from build123d import *

# Parameters (mm, degrees)
F0_W      = 150
F0_H      = 19
F1_DEPTH  = 50
F3_DEPTH  = 19
F4_W      = 79
F4_H      = 30
F5_DEPTH  = 35.4
F8_DEPTH  = 30
F9_W      = 54.530326277
F9_H      = 30
F10_DEPTH = 2
F12_DEPTH = 13
F14_DEPTH = 13
F15_R     = 5
F16_DEPTH = 13
F18_DEPTH = 13
F19_R     = 10
F20_DEPTH = 19
F21_DEPTH = 19


with BuildPart() as f1:
    # F0 (on Front) → F1 (new body)
    with BuildSketch(Plane.XZ):
        with Locations((0, 1.0748035961)):
            Rectangle(F0_W, F0_H)
    extrude(amount=F1_DEPTH)

    # F2 (on face) → F3 (join)
    with BuildSketch(Plane.XY.offset(10.5748035961)):
        with BuildLine():
            Line((-75, -50), (-75, 0))
            ThreePointArc((-75, 0), (-100, -25), (-75, -50))
        make_face()
        with BuildLine():
            ThreePointArc((75, -50), (100, -25), (75, 0))
            Line((75, 0), (75, -50))
        make_face()
    extrude(amount=-F3_DEPTH)

    # F4 (on Top) → F5 (join)
    with BuildSketch(Plane.XY):
        with Locations((3.0394736677, -23.589033746)):
            Rectangle(F4_W, F4_H)
    extrude(amount=F5_DEPTH)

    # F7 (on face) → F8 (cut)
    with BuildSketch(Plane.XZ.offset(38.589033746)):
        with BuildLine():
            Line((31.6433943808, 35.2142751217), (-23.7523913383, 34.8830260336))
            ThreePointArc((-23.7523913383, 34.8830260336), (4.0825457385, 12.1303321123), (31.6433943808, 35.2142751217))
        make_face()
    extrude(amount=-F8_DEPTH, mode=Mode.SUBTRACT)

    # F9 (on face) → F10 (cut)
    with BuildSketch(Plane.XY.offset(35.4)):
        with Locations((4.4306721538, -23.589033746)):
            Rectangle(F9_W, F9_H)
    extrude(amount=-F10_DEPTH, mode=Mode.SUBTRACT)

    # F11 (on face) → F12 (join)
    with BuildSketch(Plane(origin=(-36.4605263323, 0, 0), x_dir=(0, -1, 0), z_dir=(-1, 0, 0))):
        with BuildLine():
            Line((8.589033746, 35.4), (38.589033746, 35.4))
            ThreePointArc((38.589033746, 35.4), (23.589033746, 50.4), (8.589033746, 35.4))
        make_face()
    extrude(amount=-F12_DEPTH)

    # F13 (on face) → F14 (join)
    with BuildSketch(Plane.YZ.offset(42.5394736677)):
        with BuildLine():
            Line((-38.589033746, 35.4), (-8.589033746, 35.4))
            ThreePointArc((-8.589033746, 35.4), (-23.589033746, 50.4), (-38.589033746, 35.4))
        make_face()
    extrude(amount=-F14_DEPTH)

    # F15 (on face) → F16 (cut)
    with BuildSketch(Plane.YZ.offset(42.5394736677)):
        with Locations((-23.6123930663, 39.6284162998)):
            Circle(F15_R)
    extrude(amount=-F16_DEPTH, mode=Mode.SUBTRACT)

    # F17 (on face) → F18 (cut)
    with BuildSketch(Plane.YZ.offset(-23.4605263323)):
        with BuildLine():
            Line((-21.2145990318, 35.4), (-26.3218262607, 35.4))
            ThreePointArc((-26.3218262607, 35.4), (-23.7682126462, 34.6987274289), (-21.2145990318, 35.4))
        make_face()
        with BuildLine():
            ThreePointArc((-21.2145990318, 35.4), (-19.4226362707, 37.2256795192), (-18.7682126462, 39.6987274289))
            ThreePointArc((-18.7682126462, 39.6987274289), (-26.241260556, 44.0443038045), (-26.3218262607, 35.4))
            Line((-26.3218262607, 35.4), (-21.2145990318, 35.4))
        make_face()
    extrude(amount=-F18_DEPTH, mode=Mode.SUBTRACT)

    # F19 (on face) → F20 (cut)
    with BuildSketch(Plane.XY.offset(10.5748035961)):
        with Locations((-84.4740969445, -25.0065810978)):
            Circle(F19_R)
    extrude(amount=-F20_DEPTH, mode=Mode.SUBTRACT)

    # F19 (on face) → F21 (cut)
    with BuildSketch(Plane.XY.offset(10.5748035961)):
        with Locations((-84.4740969445, -25.0065810978)):
            Circle(F19_R)
        with Locations((84.4793568792, -25.0065810978)):
            Circle(F19_R)
    extrude(amount=-F21_DEPTH, mode=Mode.SUBTRACT)


solid = f1.part
Verification items for the finished model (mm, model axes). A direction names the side the tool comes from. Coordinates: 2 decimals unless noted, no trailing zeros. Order: outer loops, then holes, each group sorted by start corner. A loop starts at its lowest first (then second) coordinate and runs counter-clockwise, first axis right, second up. Notation, with made-up numbers: M 64.25,81.25 L 104.25,81.25 A15 cw 104.25,100.25 Z; hole C 58.5,86 d8. An arc over 180 degrees is marked long. Return JSON: item names as keys, results as strings.
1) Thickness scan on L1, parallel to X at y = -33, z = -2.5; L2, parallel to X at y = -24, z = -0.5; L3, parallel to X at y = -38, z = 39. Record the ranges inside material, lowest first. Write a range as [from, to].
Answer list:
{"L1": "[-98.69, -90.48], [-78.47, 78.47], [90.49, 98.69]", "L2": "[-99.98, -94.42], [-74.52, 74.53], [94.43, 99.98]", "L3": "[-36.46, -23.46], [29.54, 42.54]"}
2) Gauge pin test, flat ends, axial feed: pin 1 (0.5 mm diameter, centred on x = 31.5, y = -25, fed in from +Z) (3 decimals); pin 2 (12 mm diameter, centred on x = 84.48, y = -25.01, fed in from +Z); pin 3 (1.5 mm diameter, centred on y = -18, z = 43.5, fed in from -X); pin 4 (13 mm diameter, centred on y = -23.61, z = 39.63, fed in from +X). Record the tip position at first contact, or that the pin passes through.
Answer list:
{"pin 1": "z = 50.355", "pin 2": "through", "pin 3": "x = -36.46", "pin 4": "x = 42.54"}
3) Cross-section at C-C, the plane x = 83. Record the boundary of the cut face in (y, z), and give its area (3 significant figures).
Answer list:
{"outline": "M -48.69,-8.43 L -34.9,-8.43 L -34.9,10.57 L -48.69,10.57 Z; M -15.12,-8.43 L -1.31,-8.43 L -1.31,10.57 L -15.12,10.57 Z", "area": "524 mm2"}
4) Release check for a two-part mould opening along X. For faces 1 (the flat face through (2, -38.589, 12)), 2 (the flat face through (29.539, -24, 45)), 3 (the flat face through (42.539, -24, 31)) record: +X half, -X half, draft (parallel to the pull), parting line (faces both ways), or undercut.
Answer list:
{"face 1": "draft", "face 2": "undercut", "face 3": "+X half"}
5) Access from +Z, -Z, +X, -X, +Y, -Y to the whole of each face (thin tool, end or side, straight path). Record for faces 4 (the flat face through (-36.461, -23, 31)), 5 (the cylindrical face through (36.13, -24.263, 44.586)), 6 (the flat face through (2, -8.589, 12)).
Answer list:
{"face 4": "+Z, -X, +Y, -Y", "face 5": "+X", "face 6": "+Z, +X, -X, +Y"}
6) Cross-section at D-D, the plane y = -13. Record the boundary of the cut face in (x, z).
Answer list:
{"outline": "M -96.93,-8.43 L 96.93,-8.43 L 96.93,10.57 L 42.54,10.57 L 42.54,46.02 L 29.54,46.02 L 29.54,35.4 L 31.7,35.4 L 31.7,33.4 L 31.25,33.4 A28.2 cw -23.75,34.88 L -22.83,34.89 L -22.83,35.4 L -23.46,35.4 L -23.46,46.02 L -36.46,46.02 L -36.46,10.57 L -96.93,10.57 Z"}
7) Cross-section at B-B, the plane z = 25.5. Record the boundary of the cut face in (x, y).
Answer list:
{"outline": "M -36.46,-38.59 L -20.07,-38.59 L -20.07,-8.59 L -36.46,-8.59 Z; M 27.9,-38.59 L 42.54,-38.59 L 42.54,-8.59 L 27.9,-8.59 Z"}
8) Cross-section at A-A, the plane x = -30. Record the boundary of the cut face in (y, z).
Answer list:
{"outline": "M -50,-8.43 L 0,-8.43 L 0,10.57 L -8.59,10.57 L -8.59,35.4 A15 ccw -38.59,35.4 L -38.59,10.57 L -50,10.57 Z; hole C -23.77,39.7 d10"}
